Here's the drawing with two shaded views (mm, measured from the low corner). I have some questions. A direction names the side the tool comes from. Round coordinates to 2 decimals unless told otherwise and drop trailing zeros. Loops run counter-clockwise (first coordinate to the right, second up) from the corner with the lowest first, then second, coordinate; pieces in that order, holes last. Notation, with made-up numbers: M 6.25,26 L 11.25,26 A28 cw 11.25,64 Z; hole C 88.5,-27.75 d7. An arc over 180 degrees is marked long. Answer as a JSON object with one key per item and string values.
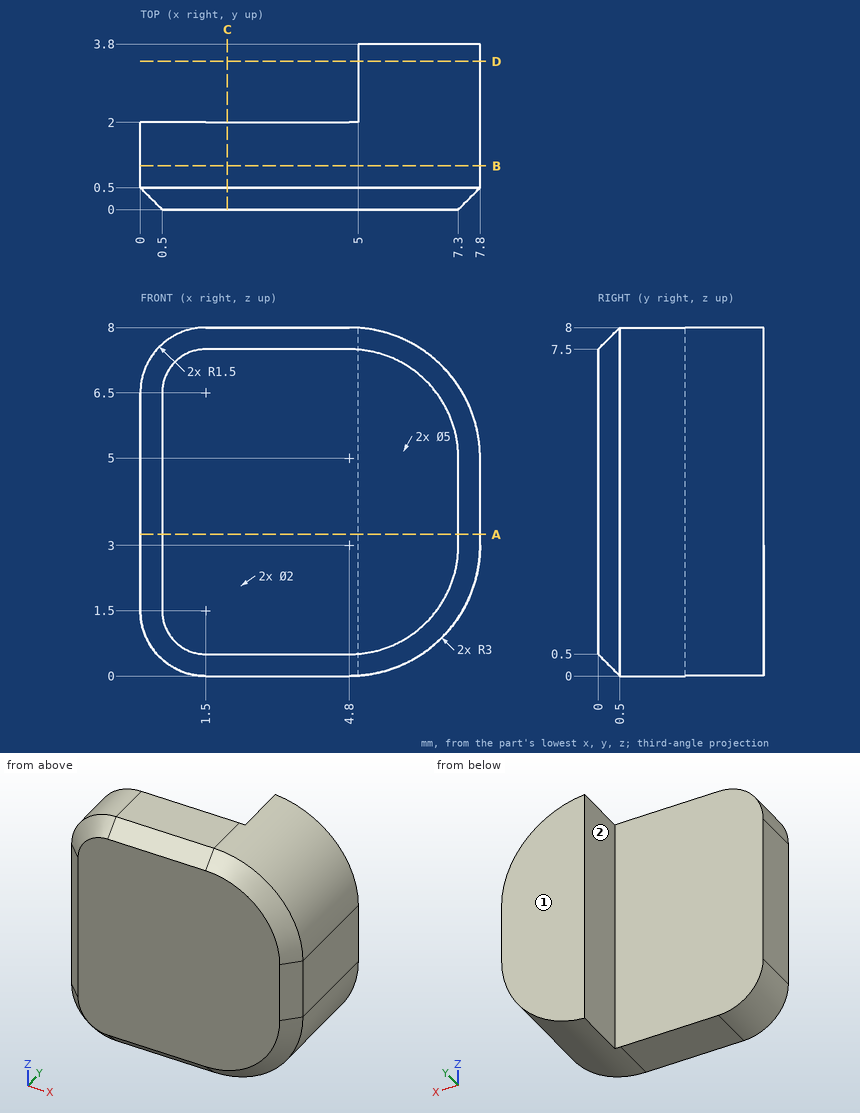
Item 1: For the marked faces 1 and 2, which set-ups out of +Z, -Z, +X, -X, +Y, -Y let a thin tool reach every point of the face, with its end or its side?
Solution:
{"face 1": "+Z, -Z, +X, -X, +Y", "face 2": "+Z, -Z, -X, +Y"}
Item 2: I want a section at D-D on y = 3.4. List the corners of the cut face in (x, z) for me.
Solution:
{"outline": "M 5,0.01 A3 ccw 7.8,3 L 7.8,5 A3 ccw 5,7.99 Z"}
Item 3: I want a section at B-B on y = 1. List the corners of the cut face in (x, z) for me.
Solution:
{"outline": "M 0,1.5 A1.5 ccw 1.5,0 L 4.8,0 A3 ccw 7.8,3 L 7.8,5 A3 ccw 4.8,8 L 1.5,8 A1.5 ccw 0,6.5 Z"}
Item 4: I want a section at A-A on z = 3.25. List the corners of the cut face in (x, y) for me.
Solution:
{"outline": "M 0,0.5 L 0.5,0 L 7.3,0 L 7.8,0.5 L 7.8,3.8 L 5,3.8 L 5,2 L 0,2 Z"}
Item 5: If I drill on L1, parallel to Y at x = 2.5, z = 2.75; L2, parallel to Z at x = 5, y = 0.85; L3, parallel to X at y = 2.8, z = 5, over which ranges is the centre line in solid material (lowest first)? Write a range as from..to.
Solution:
{"L1": "y = 0..2", "L2": "z = 0.01..7.99", "L3": "x = 5..7.8"}
Item 6: For P1, Ø1.5, axis at x = 2, z = 2.5, coming from the +Y side; P2, Ø4, axis at x = 4, z = 1.5, coming from the -Y side; P3, Ø0.9, axis at y = 3, z = 4, coming from the -X side, each with a flat end and sliding along its axis, tell me the tip position at first contact or that it passes through.
Solution:
{"P1": "stops at y = 2", "P2": "stops at y = 0", "P3": "stops at x = 5"}
Item 7: I want a section at C-C on x = 2. List the corners of the cut face in (y, z) for me.
Solution:
{"outline": "M 0,0.5 L 0.5,0 L 2,0 L 2,8 L 0.5,8 L 0,7.5 Z"}
